For this review, take the finished solid that the model builds, in its own axes (mm). A direction names the side the tool comes from. Coordinates: 2 decimals unless noted, no trailing zeros. Order: outer loops, then holes, each group sorted by start corner. A loop starts at its lowest first (then second) coordinate and runs counter-clockwise, first axis right, second up. Notation, with made-up numbers: (65.25, -9) -> (74.25, -9) arc R17 cw to (74.25, 19) -> close; hole circle Ø3 at (-24, -22.75). An arc over 180 degrees is marked (long way). Answer as a JSON object with one key per item and string values. Group by question number.
1) Draft analysis for pull direction X (two halves, no side actions). For faces 1 (the flat face through (-20, 18, 11)), 2 (the flat face through (-23, -18.31, -14)), 3 (the cylindrical face through (10.86, 18.1, 11.24)), 4 (the flat face through (10, 10, 11)), state which applies: +X half, -X half, draft (parallel to the pull), parting line (faces both ways), or undercut.
2) Add section B-B, the plane x = 0. Write out the cut boundary in (y, z).
3) Add section C-C, the plane y = -15.5. Write out the cut boundary in (x, z), then the cut area to 3 significant figures.
4) Add section D-D, the plane z = 8.5. Write out the cut boundary in (x, y), then the cut area to 3 significant figures.
5) For pin 1 (2 mm diameter, centred on x = 16.5, z = -4.5, fed in from +Y); pin 2 (1.2 mm diameter, centred on y = 1.5, z = 11, fed in from +X); pin 3 (7.5 mm diameter, centred on x = 12, z = -1, fed in from -Y), all flat-tipped, find the tip position at first contact; note any pin that passes through.
6) Wall thickness on L1, parallel to Y at x = -15.5, z = 10.7; L2, parallel to X at y = -10.5, z = -37; L3, parallel to Y at x = 15, z = 11: over which ranges is each line inside the solid? List them lowest first.
7) Machinability: for faces 5 (the cylindrical face through (11.04, -0.07, 11.07)), 6 (the flat face through (-19, -19, -15)), 7 (the flat face through (12, -28.31, -13)), which of the approach directions +Z, -Z, +X, -X, +Y, -Y give a long, thin tool a straight path to every point of the face, cutting with its end or side? Answer none if there is none.
8) Add section A-A, the plane y = 1. Write out the cut boundary in (x, z), then the cut area to 3 significant figures.
from build123d import *

# Parameters (mm, degrees)
PAD021_DEPTH    = 2.45
PAD022_DEPTH    = 50
SKETCH044_R     = 1.5
POCKET019_DEPTH = 5
SKETCH045_W     = 20
SKETCH045_H     = 52.45
PAD023_DEPTH    = 1
POCKET020_DEPTH = 3
SKETCH047_W     = 26
SKETCH047_H     = 52.45
PAD024_DEPTH    = 6.46
SKETCH048_W     = 17
SKETCH048_H     = 52.45
PAD025_DEPTH    = 3.31
SKETCH049_W     = 1
SKETCH049_H     = 52.45
PAD026_DEPTH    = 3.31
FILLET002_R     = 2
FILLET003_R     = 2
SKETCH050_W     = 10
SKETCH050_H     = 52.45
PAD027_DEPTH    = 5
FILLET004_R     = 2
SKETCH051_R     = 11.04
POCKET021_DEPTH = 5
SKETCH052_R     = 11.04
POCKET022_DEPTH = 5
SKETCH053_R     = 16.5
PAD028_DEPTH    = 0.35
SKETCH054_W     = 20
SKETCH054_H     = 31.6
POCKET023_DEPTH = 5
SKETCH055_R     = 11.04
POCKET024_DEPTH = 5
FILLET005_R     = 3
FILLET006_R     = 0.5


with BuildPart() as part:
    # Sketch041 → Pad021 (new body)
    with BuildSketch(Plane.XY):
        Polygon((-21, 22), (-10, 22), (-10, -8), (10, -8), (10, 22), (21, 22), (21, -22), (-21, -22), align=None)
    extrude(amount=PAD021_DEPTH)

    # Sketch043 (on Face9 of Pad021) → Pad022 (join)
    with BuildSketch(Plane(origin=(0, 0, 0), x_dir=(1, 0, 0), z_dir=(0, 0, -1))):
        Polygon((21, 14), (21, 22), (-21, 22), (-21, 14), (-17, 18), (17, 18), align=None)
    extrude(amount=PAD022_DEPTH)

    # Sketch044 (on Face4 of Pad022) → Pocket019 (cut)
    with BuildSketch(Plane.XY.offset(2.45)):
        with Locations((-15.5, 18.5)):
            Circle(SKETCH044_R)
        with Locations((-15.5, -12.5)):
            Circle(SKETCH044_R)
    pocket019 = extrude(amount=-POCKET019_DEPTH, mode=Mode.SUBTRACT)

    # Mirrored: Pocket019 across Sketch044 V_Axis
    add(pocket019.mirror(Plane(origin=(0, 0, 2.45), x_dir=(0, 0, 1), z_dir=(1, 0, 0))), mode=Mode.SUBTRACT)

    # Sketch045 (on Face13 of Mirrored) → Pad023 (join)
    with BuildSketch(Plane(origin=(-21, 0, 0), x_dir=(0, -1, 0), z_dir=(-1, 0, 0))):
        with Locations((12, -23.775)):
            Rectangle(SKETCH045_W, SKETCH045_H)
    pad023 = extrude(amount=PAD023_DEPTH)

    # Mirrored024: Pad023 across YZ
    add(pad023.mirror(Plane.YZ))

    # Sketch046 (on Face22 of Mirrored024) → Pocket020 (cut)
    with BuildSketch(Plane.XY.offset(2.45)):
        Polygon((-21, 20), (-13.23582, 27.76418), (-21, 27.957458), align=None)
    pocket020 = extrude(amount=-POCKET020_DEPTH, mode=Mode.SUBTRACT)

    # Mirrored025: Pocket020 across Sketch046 V_Axis
    add(pocket020.mirror(Plane(origin=(0, 0, 2.45), x_dir=(0, 0, 1), z_dir=(1, 0, 0))), mode=Mode.SUBTRACT)

    # Sketch047 (on Face13 of Pad022) → Pad024 (join)
    with BuildSketch(Plane.XZ.offset(22)):
        with Locations((-8, -23.775)):
            Rectangle(SKETCH047_W, SKETCH047_H)
    extrude(amount=PAD024_DEPTH)

    # Sketch048 (on Face22 of Pad024) → Pad025 (join)
    with BuildSketch(Plane.XZ.offset(22)):
        with Locations((13.5, -23.775)):
            Rectangle(SKETCH048_W, SKETCH048_H)
    extrude(amount=PAD025_DEPTH)

    # Sketch049 (on Face22 of Pad025) → Pad026 (join)
    with BuildSketch(Plane.XZ.offset(22)):
        with Locations((-21.5, -23.775)):
            Rectangle(SKETCH049_W, SKETCH049_H)
    extrude(amount=PAD026_DEPTH)

    # Fillet002
    fillet002_edges = [part.edges().sort_by_distance(p)[0] for p in [
        (5, -28.46, -23.775),
        (22, -25.31, -23.775),
    ]]
    fillet(fillet002_edges, radius=FILLET002_R)

    # Fillet003
    fillet003_edges = [part.edges().sort_by_distance(p)[0] for p in [
        (-21, -28.46, -23.775),
    ]]
    fillet(fillet003_edges, radius=FILLET003_R)

    # Sketch050 (on Face10 of Fillet003) → Pad027 (join)
    with BuildSketch(Plane(origin=(-22, 0, 0), x_dir=(0, -1, 0), z_dir=(-1, 0, 0))):
        with Locations((20.31, -23.775)):
            Rectangle(SKETCH050_W, SKETCH050_H)
    extrude(amount=PAD027_DEPTH)

    # Fillet004
    fillet004_edges = [part.edges().sort_by_distance(p)[0] for p in [
        (-27, -25.31, -23.775),
        (-27, -15.31, -23.775),
    ]]
    fillet(fillet004_edges, radius=FILLET004_R)

    # Sketch051 (on Face37 of Fillet004) → Pocket021 (cut)
    with BuildSketch(Plane(origin=(0, 0, 0), x_dir=(1, 0, 0), z_dir=(0, 0, -1))):
        with Locations((0, -3)):
            Circle(SKETCH051_R)
    extrude(amount=-POCKET021_DEPTH, mode=Mode.SUBTRACT)

    # Sketch052 (on Face28 of Pad027) → Pocket022 (cut)
    with BuildSketch(Plane(origin=(0, 0, 0), x_dir=(1, 0, 0), z_dir=(0, 0, -1))):
        with Locations((0, -3)):
            Circle(SKETCH052_R)
    extrude(amount=-POCKET022_DEPTH, mode=Mode.SUBTRACT)

    # Sketch053 (on Face42 of Pocket022) → Pad028 (join)
    with BuildSketch(Plane(origin=(0, 0, 0), x_dir=(1, 0, 0), z_dir=(0, 0, -1))):
        with Locations((0, -3)):
            Circle(SKETCH053_R)
    extrude(amount=PAD028_DEPTH)

    # Sketch054 (on Face44 of Pad028) → Pocket023 (cut)
    with BuildSketch(Plane.XY):
        with Locations((0, 7.8)):
            Rectangle(SKETCH054_W, SKETCH054_H)
    extrude(amount=-POCKET023_DEPTH, mode=Mode.SUBTRACT)

    # Sketch055 (on Face5 of Pocket023) → Pocket024 (cut)
    with BuildSketch(Plane.XY.offset(2.45)):
        with Locations((0, 3)):
            Circle(SKETCH055_R)
    extrude(amount=-POCKET024_DEPTH, mode=Mode.SUBTRACT)

    # Fillet005
    fillet005_edges = [part.edges().sort_by_distance(p)[0] for p in [
        (-10, 22, 1.225),
        (10, 22, 1.225),
    ]]
    fillet(fillet005_edges, radius=FILLET005_R)

    # Fillet006
    fillet006_edges = [part.edges().sort_by_distance(p)[0] for p in [
        (22, -2, -23.775),
        (-22, -2, -23.775),
    ]]
    fillet(fillet006_edges, radius=FILLET006_R)


with BuildPart() as part_1:
    # Body006 placement: moved
    add(part.part.moved(Location((0, -3, 10))))


solid = part_1.part
Output values:
{
 "1": {"face 1": "-X half", "face 2": "draft", "face 3": "undercut", "face 4": "undercut"},
 "2": {"outline": "(-31.46, -40) -> (-21, -40) -> (-21, 10) -> (-16.5, 10) -> (-16.5, 9.65) -> (-11.04, 9.65) -> (-11.04, 12.45) -> (-31.46, 12.45) -> close"},
 "3": {"outline": "(-22, -40) -> (-21, -40) -> (-21, 10) -> (-17, 10) -> (-17, 12.45) -> (-22, 12.45) -> close; (-14, 10) -> (-5.66, 10) -> (-5.66, 9.65) -> (5.66, 9.65) -> (5.66, 10) -> (14, 10) -> (14, 12.45) -> (-14, 12.45) -> close; (17, 10) -> (21, 10) -> (21, -40) -> (22, -40) -> (22, 12.45) -> (17, 12.45) -> close", "area": "197 mm²"},
 "4": {"outline": "(-27, -26.31) arc R2 ccw to (-25, -28.31) -> (-21, -28.31) -> (-21, -29.46) arc R2 ccw to (-19, -31.46) -> (3, -31.46) arc R2 ccw to (5, -29.46) -> (5, -28.31) -> (20, -28.31) arc R2 ccw to (22, -26.31) -> (22, -5.5) arc R0.5 ccw to (21.5, -5) -> (21, -5) -> (21, -17) -> (17, -21) -> (-17, -21) -> (-21, -17) -> (-21, -5) -> (-21.5, -5) arc R0.5 ccw to (-22, -5.5) -> (-22, -18.31) -> (-25, -18.31) arc R2 ccw to (-27, -20.31) -> close", "area": "497 mm²"},
 "5": {"pin 1": "stops at y = -20.5", "pin 2": "stops at x = 21", "pin 3": "stops at y = -28.31"},
 "6": {"L1": "y = -31.46 to -17, -14 to 14, 17 to 19", "L2": "x = -22 to -21, 21 to 22", "L3": "y = -28.31 to -16.91, -14.09 to 14.09, 16.91 to 19"},
 "7": {"face 5": "+Z, -Z", "face 6": "-Z, +Y", "face 7": "+Z, -Z, +X, -Y"},
 "8": {"outline": "(-21, 10) -> (-16.47, 10) -> (-16.47, 9.65) -> (-10.99, 9.65) -> (-10.99, 12.45) -> (-21, 12.45) -> close; (10.99, 9.65) -> (16.47, 9.65) -> (16.47, 10) -> (21, 10) -> (21, 12.45) -> (10.99, 12.45) -> close", "area": "52.9 mm²"}
}
